Could you check a few things on this model? Use its own coordinates, in mm. A direction names the side the tool comes from. Coordinates: 2 decimals unless noted, no trailing zeros. Order: outer loops, then holes, each group sorted by start corner. A loop starts at its lowest first (then second) coordinate and runs counter-clockwise, first axis right, second up. Notation, with made-up numbers: (37, 66.5) -> (82, 66.5) arc R3 cw to (82, 70.5) -> close; hole circle Ø8 at (12.25, 83.25). An arc over 180 degrees is marked (long way). Put each result on its own line as item: value. Start each with the question number.
Q1. If we section it at A-A (z = -18): Please give me the cut outline in (x, y), and give its area (3 significant figures).
Q2. For faces 4 (the face through (-4.05, -28.73, -12.71)), 5 (the face through (1, 11.754, -5)), 6 (the face through (-1, 6, 16)), which set-ups out of +Z, -Z, +X, -X, +Y, -Y let a thin tool reach every point of the face, with its end or its side?
Q3. We'd pull the mould along Y, two halves only. Please class faces 1 (the face through (3.81, -5, -5)), 2 (the face through (-3, -8, 7.427)), 3 (the face through (-4, -4.382, 4)): +Y half, -Y half, draft (parallel to the pull), parting line (faces both ways), or undercut.
Q4. Will these pins go through, and if not, where does the flat tip stop? pin 1 (6 mm diameter, centred on x = 4.5, y = -16.5, fed in from -Z); pin 2 (0.8 mm diameter, centred on x = -1, y = -20.5, fed in from +Z); pin 3 (3 mm diameter, centred on y = -16.5, z = -6, fed in from -X).
Q5. If we section it at B-B (z = -12.5): Please give me the cut outline in (x, y) (3 decimals).
Q6. If we section it at D-D (y = -21.5): Please give me the cut outline in (x, z).
Q7. If we section it at C-C (y = -6.5): Please give me the cut outline in (x, z) (3 decimals).
Q8. Please list where these lines run through material, in increasing order: line 1 along X through (y, z) = (-19, -7); line 2 along Z through (x, y) = (2, -18.5); line 3 along Z through (x, y) = (1, 5.5).
from build123d import *

# Parameters (mm, degrees)
F1_DEPTH  = 6.35
F3_DEPTH  = 2.54
F5_DEPTH  = 2.54
F6_W      = 4.75
F6_H      = 6.1595766147
F8_W      = 4.75
F8_H      = 6.1471766147
F7_W      = 4.75
F7_H      = 6.1471766147
F9_W      = 4.75
F9_H      = 6.1471766147
F10_DEPTH = 6
F11_R     = 1.5
F12_R     = 1.5
F13_R     = 1.5
F14_R     = 1.5
F15_DEPTH = 6
F16_R     = 0.5
F17_DEPTH = 3.5


# Not quite as in the source:
# - a feature names something its author has since deleted; it is built from what else it names


with BuildPart() as f1:
    # F0 (on Right) → F1 (new body, symmetric)
    with BuildSketch(Plane.YZ):
        Polygon((10.3821327425, 24.0797383321), (1.8821327425, 24.0797383321), (1, 19.0769149468), (0, 19.0769149468), (0, 12.6797383321), (-8.5, 12.6797383321), (-9.3821327425, 7.6769149468), (-10.3821327425, 7.6769149468), (-10.3821327425, 1.2797383321), (-18.8821327425, 1.2797383321), (-19.7642654851, -3.7230850532), (-20.7642654851, -3.7230850532), (-20.7642654851, -10.1202616679), (-29.2642654851, -10.1202616679), (-30.1463982276, -15.1230850532), (-31.1463982276, -15.1230850532), (-31.1463982276, -23.9202616679), (11.7536017724, -23.9202616679), (11.7536017724, 14.9208800867), align=None)
    extrude(amount=F1_DEPTH, both=True)

    # F2 (on face) → F3 (cut)
    with BuildSketch(Plane(origin=(-6.35, 0, 0), x_dir=(0, -1, 0), z_dir=(-1, 0, 0))):
        Polygon((-11.7536017724, -23.9202616679), (0, -23.9202616679), (0, 12.6797383321), (0, 19.0769149468), (-1, 19.0769149468), (-1.8821327425, 24.0797383321), (-10.3821327425, 24.0797383321), (-11.7536017724, 14.9208800867), align=None)
        Polygon((20.7642654851, -23.9202616679), (20.7642654851, -10.1202616679), (20.7642654851, -3.7230850532), (19.7642654851, -3.7230850532), (18.8821327425, 1.2797383321), (10.3821327425, 1.2797383321), (10.3821327425, -23.9202616679), align=None)
    extrude(amount=-F3_DEPTH, mode=Mode.SUBTRACT)

    # F4 (on face) → F5 (cut)
    with BuildSketch(Plane.YZ.offset(6.35)):
        Polygon((-20.7642654851, -23.9202616679), (-20.7642654851, -10.1202616679), (-29.2642654851, -10.1202616679), (-30.1463982276, -15.1230850532), (-31.1463982276, -15.1230850532), (-31.1463982276, -23.9202616679), align=None)
        Polygon((-10.3821327425, 1.2797383321), (-10.3821327425, -23.9202616679), (0, -23.9202616679), (0, 12.6797383321), (-8.5, 12.6797383321), (-9.3821327425, 7.6769149468), (-10.3821327425, 7.6769149468), align=None)
    extrude(amount=-F5_DEPTH, mode=Mode.SUBTRACT)

    # F6 (on face) + F8 (on face) + F7 (on face) + F9 (on face) → F10 (cut)
    with BuildSketch(Plane.XZ.offset(31.1463982276)):
        with Locations((-3.725, -18.4528733606)):
            Rectangle(F6_W, F6_H)
        with Locations((1.275, -18.4528733606)):
            Rectangle(F6_W, F6_H)
        with Locations((6.275, -18.4528733606)):
            Rectangle(F6_W, F6_H)
    with BuildSketch(Plane.XZ.offset(10.3821327425)):
        Polygon((-6.1, 7.4269149468), (-6.1, 1.2797383321), (-3.81, 1.2797383321), (-1.35, 1.2797383321), (-1.35, 7.4269149468), align=None)
        with Locations((1.275, 4.3533266394)):
            Rectangle(F8_W, F8_H)
        with Locations((6.275, 4.3533266394)):
            Rectangle(F8_W, F8_H)
    with BuildSketch(Plane.XZ.offset(20.7642654851)):
        with Locations((-1.185, -7.0466733606)):
            Rectangle(F7_W, F7_H)
        Polygon((1.44, -3.9730850532), (1.44, -10.1202616679), (3.81, -10.1202616679), (6.19, -10.1202616679), (6.19, -3.9730850532), align=None)
        with Locations((8.815, -7.0466733606)):
            Rectangle(F7_W, F7_H)
    with BuildSketch(Plane.XZ):
        with Locations((-1.185, 15.7533266394)):
            Rectangle(F9_W, F9_H)
        Polygon((1.44, 18.8269149468), (1.44, 12.6797383321), (3.81, 12.6797383321), (6.19, 12.6797383321), (6.19, 18.8269149468), align=None)
        with Locations((8.815, 15.7533266394)):
            Rectangle(F9_W, F9_H)
    extrude(amount=-F10_DEPTH, mode=Mode.SUBTRACT)

    # F11 (on face) + F12 (on face) + F13 (on face) + F14 (on face) → F15 (cut)
    with BuildSketch(Plane.XY.offset(-10.1202616679)):
        with Locations((-3.725, -27.2642654851)):
            Circle(F11_R)
        with Locations((1.275, -27.2642654851)):
            Circle(F11_R)
        with Locations((6.275, -27.2642654851)):
            Circle(F11_R)
    with BuildSketch(Plane.XY.offset(1.2797383321)):
        with Locations((-1.185, -16.8821327425)):
            Circle(F12_R)
        with Locations((3.815, -16.8821327425)):
            Circle(F12_R)
        with Locations((8.815, -16.8821327425)):
            Circle(F12_R)
    with BuildSketch(Plane.XY.offset(12.6797383321)):
        with Locations((-3.725, -6.5)):
            Circle(F13_R)
        with Locations((1.275, -6.5)):
            Circle(F13_R)
        with Locations((6.275, -6.5)):
            Circle(F13_R)
    with BuildSketch(Plane.XY.offset(24.0797383321)):
        with Locations((-1.185, 3.8821327425)):
            Circle(F14_R)
        with Locations((3.815, 3.8821327425)):
            Circle(F14_R)
        with Locations((8.815, 3.8821327425)):
            Circle(F14_R)
    extrude(amount=-F15_DEPTH, mode=Mode.SUBTRACT)

    # F16 (on face) → F17 (join)
    with BuildSketch(Plane(origin=(0, 0, -23.9202616679), x_dir=(1, 0, 0), z_dir=(0, 0, -1))):
        with Locations((1.27, 26.4963982276)):
            Circle(F16_R)
        with Locations((-3.81, 26.4963982276)):
            Circle(F16_R)
        with Locations((3.81, 11.2563982276)):
            Circle(F16_R)
        with Locations((-1.27, 11.2563982276)):
            Circle(F16_R)
        with Locations((-3.81, 1.0963982276)):
            Circle(F16_R)
        with Locations((1.27, 1.0963982276)):
            Circle(F16_R)
        with Locations((3.81, -9.0636017724)):
            Circle(F16_R)
        with Locations((-1.27, -9.0636017724)):
            Circle(F16_R)
    extrude(amount=F17_DEPTH)


solid = f1.part
The answers:
1. outline: (-6.35, -31.15) -> (-6.1, -31.15) -> (-6.1, -25.15) -> (-1.35, -25.15) -> (-1.35, -31.15) -> (-1.1, -31.15) -> (-1.1, -25.15) -> (3.65, -25.15) -> (3.65, -31.15) -> (3.81, -31.15) -> (3.81, -20.76) -> (6.35, -20.76) -> (6.35, -10.38) -> (3.81, -10.38) -> (3.81, 0) -> (6.35, 0) -> (6.35, 11.75) -> (-3.81, 11.75) -> (-3.81, 0) -> (-6.35, 0) -> (-6.35, -10.38) -> (-3.81, -10.38) -> (-3.81, -20.76) -> (-6.35, -20.76) -> close
1. area: 379 mm^2
2. face 4: +Z
2. face 5: +Z, -Z, +X, -X, +Y
2. face 6: -Y
3. face 1: undercut
3. face 2: draft
3. face 3: -Y half
4. pin 1: z = -23.92
4. pin 2: z = -3.72
4. pin 3: x = -3.81
5. outline: (-6.35, -29.684) -> (3.81, -29.684) -> (3.81, -20.764) -> (6.35, -20.764) -> (6.35, -10.382) -> (3.81, -10.382) -> (3.81, 0) -> (6.35, 0) -> (6.35, 11.754) -> (-3.81, 11.754) -> (-3.81, 0) -> (-6.35, 0) -> (-6.35, -10.382) -> (-3.81, -10.382) -> (-3.81, -20.764) -> (-6.35, -20.764) -> close; hole circle Ø3 at (-3.725, -27.264); hole circle Ø3 at (1.275, -27.264)
6. outline: (-6.35, -23.92) -> (3.81, -23.92) -> (3.81, -10.12) -> (-6.35, -10.12) -> close
7. outline: (-6.35, -23.92) -> (3.81, -23.92) -> (3.81, 12.68) -> (2.775, 12.68) -> (2.775, 7.427) -> (3.65, 7.427) -> (3.65, 1.28) -> (-1.1, 1.28) -> (-1.1, 7.427) -> (-0.225, 7.427) -> (-0.225, 12.68) -> (-2.225, 12.68) -> (-2.225, 7.427) -> (-1.35, 7.427) -> (-1.35, 1.28) -> (-6.1, 1.28) -> (-6.1, 7.427) -> (-5.225, 7.427) -> (-5.225, 12.68) -> (-6.35, 12.68) -> close
8. line 1: -3.81 to -3.56, 1.19 to 1.44, 6.19 to 6.35
8. line 2: -23.92 to -10.12, -3.97 to 1.28
8. line 3: -23.92 to 12.68, 18.83 to 24.08
